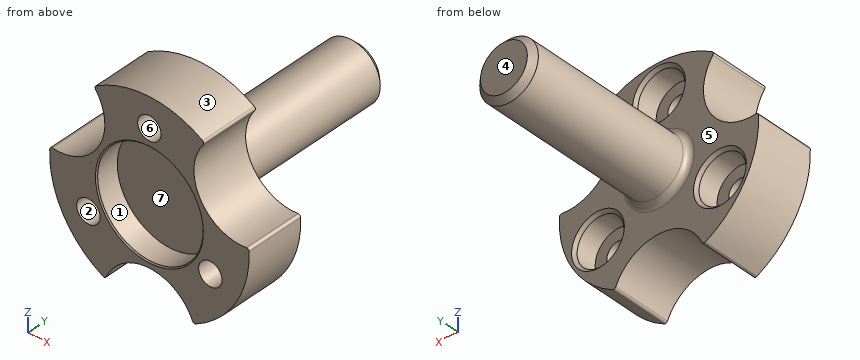
from build123d import *

# Parameters (mm, degrees)
CUT_EXTRUDE1_REACH = 25.335
SKETCH2_R          = 4
SKETCH2_R_2        = 1
FILLET1_R          = 0.2
SKETCH3_R          = 2
CUT_EXTRUDE2_DEPTH = 2
CHAMFER1_SIZE      = 0.25


with BuildPart() as part:
    # Sketch1 → Revolve1 (revolve)
    with BuildSketch(Plane.XY, mode=Mode.PRIVATE) as revolve1_sk:
        with BuildLine():
            Line((4.6, 0), (8.5, 0))
            Line((8.5, 0), (8.5, 5))
            Line((8.5, 5), (3, 5))
            ThreePointArc((3, 5), (2.646446609, 5.146446609), (2.5, 5.5))
            Line((2.5, 5.5), (2.5, 19.5))
            Line((2.5, 19.5), (2, 20))
            Line((2, 20), (0, 20))
            Line((0, 20), (0, 2))
            Line((0, 2), (4.5, 2))
            Line((4.5, 2), (4.5, 0.1))
            Line((4.5, 0.1), (4.6, 0))
        make_face()
    revolve(revolve1_sk.sketch.rotate(Axis((0, 20, 0), (0, -1, 0)), 90), axis=Axis((0, 20, 0), (0, -1, 0)))

    # Sketch2 → Cut-Extrude1 (cut, up to next)
    with BuildSketch(Plane.XZ, mode=Mode.PRIVATE) as cut_extrude1_sk1:
        with Locations((7.794228634, 4.5)):
            Circle(SKETCH2_R)
    cut_extrude1_tool1 = extrude(cut_extrude1_sk1.sketch, amount=-CUT_EXTRUDE1_REACH, mode=Mode.PRIVATE) & part.part
    # Sketch2 → Cut-Extrude1 (cut, up to next)
    with BuildSketch(Plane.XZ, mode=Mode.PRIVATE) as cut_extrude1_sk2:
        with Locations(Location((0, 6, 0), (0, 0, 270))):
            Circle(SKETCH2_R_2)
    cut_extrude1_tool2 = extrude(cut_extrude1_sk2.sketch, amount=-CUT_EXTRUDE1_REACH, mode=Mode.PRIVATE) & part.part
    # Sketch2 → Cut-Extrude1 (cut, up to next)
    with BuildSketch(Plane.XZ, mode=Mode.PRIVATE) as cut_extrude1_sk3:
        with Locations(Location((5.196152423, -3, 0), (0, 0, 270))):
            Circle(SKETCH2_R_2)
    cut_extrude1_tool3 = extrude(cut_extrude1_sk3.sketch, amount=-CUT_EXTRUDE1_REACH, mode=Mode.PRIVATE) & part.part
    # Sketch2 → Cut-Extrude1 (cut, up to next)
    with BuildSketch(Plane.XZ, mode=Mode.PRIVATE) as cut_extrude1_sk4:
        with Locations((0, -9)):
            Circle(SKETCH2_R)
    cut_extrude1_tool4 = extrude(cut_extrude1_sk4.sketch, amount=-CUT_EXTRUDE1_REACH, mode=Mode.PRIVATE) & part.part
    # Sketch2 → Cut-Extrude1 (cut, up to next)
    with BuildSketch(Plane.XZ, mode=Mode.PRIVATE) as cut_extrude1_sk5:
        with Locations(Location((-5.196152423, -3, 0), (0, 0, 270))):
            Circle(SKETCH2_R_2)
    cut_extrude1_tool5 = extrude(cut_extrude1_sk5.sketch, amount=-CUT_EXTRUDE1_REACH, mode=Mode.PRIVATE) & part.part
    # Sketch2 → Cut-Extrude1 (cut, up to next)
    with BuildSketch(Plane.XZ, mode=Mode.PRIVATE) as cut_extrude1_sk6:
        with Locations((-7.794228634, 4.5)):
            Circle(SKETCH2_R)
    cut_extrude1_tool6 = extrude(cut_extrude1_sk6.sketch, amount=-CUT_EXTRUDE1_REACH, mode=Mode.PRIVATE) & part.part
    add(cut_extrude1_tool1.solids().sort_by_distance((7.794229, 0, 4.5))[0], mode=Mode.SUBTRACT)
    add(cut_extrude1_tool2.solids().sort_by_distance((0, 0, 6))[0], mode=Mode.SUBTRACT)
    add(cut_extrude1_tool3.solids().sort_by_distance((5.196152, 0, -3))[0], mode=Mode.SUBTRACT)
    add(cut_extrude1_tool4.solids().sort_by_distance((0, 0, -9))[0], mode=Mode.SUBTRACT)
    add(cut_extrude1_tool5.solids().sort_by_distance((-5.196152, 0, -3))[0], mode=Mode.SUBTRACT)
    add(cut_extrude1_tool6.solids().sort_by_distance((-7.794229, 0, 4.5))[0], mode=Mode.SUBTRACT)

    # Fillet1
    fillet1_edges = [part.edges().sort_by_distance(p)[0] for p in [
        (8.481566104, 2.5, 0.55949658),
        (4.725321304, 2.5, 7.06550342),
        (-3.7562448, 2.5, -7.625),
        (3.7562448, 2.5, -7.625),
        (-4.725321304, 2.5, 7.06550342),
        (-8.481566104, 2.5, 0.55949658),
    ]]
    fillet(fillet1_edges, radius=FILLET1_R)

    # Sketch3 → Cut-Extrude2 (cut)
    with BuildSketch(Plane(origin=(0, 5, 0), x_dir=(1, 0, 0), z_dir=(0, 1, 0))):
        with Locations(Location((0, -6, 0), (0, 0, 270))):
            Circle(SKETCH3_R)
        with Locations(Location((-5.196152423, 3, 0), (0, 0, 270))):
            Circle(SKETCH3_R)
        with Locations(Location((5.196152423, 3, 0), (0, 0, 270))):
            Circle(SKETCH3_R)
    extrude(amount=-CUT_EXTRUDE2_DEPTH, mode=Mode.SUBTRACT)

    # Chamfer1
    chamfer1_edges = [part.edges().sort_by_distance(p)[0] for p in [
        (-5.196152423, 5, -5),
        (5.196152423, 5, -5),
        (0, 5, 4),
    ]]
    chamfer(chamfer1_edges, length=CHAMFER1_SIZE)


solid = part.part
Design review of the part built by this model. Coordinates are the model's own, in mm. Face numbers are marked on the shaded views. A direction names the side the tool comes from. Round coordinates to 2 decimals unless told otherwise and drop trailing zeros. Write each loop counter-clockwise with the first axis right and the second up, starting at its lowest first coordinate (ties: lowest second). Pieces come first, ordered by that corner, then holes. Notation, with made-up numbers: (76, 78.5) -> (129, 78.5) arc R13 ccw to (129, 100.5) -> close; hole circle Ø8 at (62, 81.25). An arc over 180 degrees is marked (long way). One line per question, with ' | ' between items.
(1) Take a section at B-B, the plane z = -6. State the section outline as (x, y) points, and give its area (3 significant figures).
Result sheet:
outline: (-6.02, 0) -> (-2.65, 0) -> (-2.65, 5) -> (-6.02, 5) -> close; (2.65, 0) -> (6.02, 0) -> (6.02, 5) -> (2.65, 5) -> close | area: 33.8 mm2
(2) Take a section at C-C, the plane y = 12. State the section outline as (x, z) points, and give its area (3 significant figures).
Result sheet:
outline: circle Ø5 at (0, 0) | area: 19.6 mm2
(3) Machinability: for the marked faces 5, 6 and 7, which of the approach directions +Z, -Z, +X, -X, +Y, -Y give a long, thin tool a straight path to every point of the face, cutting with its end or side? Answer none if there is none.
Result sheet:
face 5: +Y | face 6: +Y, -Y | face 7: -Y
(4) Insertion check: P1, Ø5, axis at x = 5.2, z = -3, coming from the +Y side; P2, Ø3, axis at x = 4.5, z = -3, coming from the +Y side; P3, Ø3, axis at x = -5.2, z = -3, coming from the +Y side. Each pin has a flat end and moves straight along its axis. Give the tip position at first contact, or say it passes through.
Result sheet:
P1: y = 5 | P2: y = 4.95 | P3: y = 3
(5) Wall thickness on line 1 (X direction, y = 4.4, z = -3); line 2 (X direction, y = 1.9, z = -3); line 3 (Y direction, x = 1.75, z = 2.5): over which ranges is each line inside the solid? List them lowest first. Write a range as [from, to].
Result sheet:
line 1: [-7.95, -7.2], [-3.2, 3.2], [7.2, 7.95] | line 2: [-7.95, -6.2], [-4.2, -3.35], [3.35, 4.2], [6.2, 7.95] | line 3: [2, 5]
(6) Draft analysis for pull direction Z (two halves, no side actions). For the marked faces 1, 2, 3 and 4, state which applies: released by +Z, released by -Z, zero draft, split by the parting line, or undercut.
Result sheet:
face 1: undercut | face 2: undercut | face 3: released by +Z | face 4: zero draft
(7) Take a section at D-D, the plane z = 6. State the section outline as (x, y) points.
Result sheet:
outline: (-4.09, 0) -> (-1, 0) -> (-1, 3) -> (-2, 3) -> (-2, 4.75) -> (-2.25, 5) -> (-4.09, 5) -> close; (1, 0) -> (4.09, 0) -> (4.09, 5) -> (2.25, 5) -> (2, 4.75) -> (2, 3) -> (1, 3) -> close
(8) Take a section at A-A, the plane z = 0. State the section outline as (x, y) points.
Result sheet:
outline: (-8.5, 0) -> (-4.6, 0) -> (-4.5, 0.1) -> (-4.5, 2) -> (4.5, 2) -> (4.5, 0.1) -> (4.6, 0) -> (8.5, 0) -> (8.5, 5) -> (3, 5) arc R0.5 cw to (2.5, 5.5) -> (2.5, 19.5) -> (2, 20) -> (-2, 20) -> (-2.5, 19.5) -> (-2.5, 5.5) arc R0.5 cw to (-3, 5) -> (-8.5, 5) -> close
